```python
from build123d import *

# Parameters (mm, degrees)
EXTRUDE_1_DEPTH     = 36
SKETCH_2_R          = 1.05
CUT_EXTRUDE_1_DEPTH = 35
FILLET_1_R          = 1.5
FILLET_2_R          = 3
CUT_EXTRUDE_5_DEPTH = 50
SKETCH_5_W          = 24
SKETCH_5_H          = 86
SKETCH_5_R          = 5
EXTRUDE_2_DEPTH     = 1.5
SKETCH_6_W          = 2
SKETCH_6_H          = 6.336440046
CUT_EXTRUDE_6_DEPTH = 3.5
FILLET_3_R          = 1.5
FILLET_4_R          = 3
SKETCH_7_R          = 2.5
SKETCH_7_R_2        = 1.05
EXTRUDE_3_DEPTH     = 1.5
FILLET_5_R          = 1.5
CHAMFER_1_SIZE      = 2


with BuildPart() as part:
    # Эскиз1 → Вытянуть1 (new body)
    with BuildSketch(Plane.XY):
        Polygon((-20, 41.5), (0, 41.5), (0, 0), (36, 0), (36, 43.5), (60, 43.5), (60, 42), (37.5, 42), (37.5, -1.5), (-1.5, -1.5), (-1.5, 40), (-20, 40), align=None)
    extrude(amount=EXTRUDE_1_DEPTH)

    # Эскиз2 → Вырез-Вытянуть1 (cut)
    with BuildSketch(Plane(origin=(0, 41.5, 0), x_dir=(-1, 0, 0), z_dir=(0, 1, 0))):
        with Locations(Location((10, 5, 0), (0, 0, 90))):
            Circle(SKETCH_2_R)
        with Locations(Location((10, 31, 0), (0, 0, 90))):
            Circle(SKETCH_2_R)
    extrude(amount=-CUT_EXTRUDE_1_DEPTH, mode=Mode.SUBTRACT)

    # Скругление1
    fillet_1_edges = [part.edges().sort_by_distance(p)[0] for p in [
        (0, 0, 18),
        (36, 0, 18),
        (-1.5, 40, 18),
    ]]
    fillet(fillet_1_edges, radius=FILLET_1_R)

    # Скругление2
    fillet_2_edges = [part.edges().sort_by_distance(p)[0] for p in [
        (0, 41.5, 18),
        (37.5, -1.5, 18),
        (-1.5, -1.5, 18),
    ]]
    fillet(fillet_2_edges, radius=FILLET_2_R)

    # Эскиз4 → Вырез-Вытянуть5 (cut)
    with BuildSketch(Plane.ZY.offset(1.5)):
        Polygon((36, 0), (30.401923789, -1.5), (5.598076211, -1.5), (0, 0), (0, -9.726752533), (36, -8.93099636), align=None)
    extrude(amount=-CUT_EXTRUDE_5_DEPTH, mode=Mode.SUBTRACT)

    # Эскиз5 → Вытянуть2 (add)
    with BuildSketch(Plane(origin=(0, 43.5, 0), x_dir=(-1, 0, 0), z_dir=(0, 1, 0))):
        with Locations((-48, 18)):
            Rectangle(SKETCH_5_W, SKETCH_5_H)
        with Locations(Location((-48, -15, 0), (0, 0, 90))):
            Circle(SKETCH_5_R, mode=Mode.SUBTRACT)
        with Locations(Location((-48, 51, 0), (0, 0, 270))):
            Circle(SKETCH_5_R, mode=Mode.SUBTRACT)
    extrude(amount=-EXTRUDE_2_DEPTH)

    # Эскиз6 → Вырез-Вытянуть6 (cut)
    with BuildSketch(Plane.ZY.offset(-36)):
        with Locations((37, 42.938728947)):
            Rectangle(SKETCH_6_W, SKETCH_6_H)
        with Locations((-1, 42.938728947)):
            Rectangle(SKETCH_6_W, SKETCH_6_H)
    extrude(amount=-CUT_EXTRUDE_6_DEPTH, mode=Mode.SUBTRACT)

    # Скругление3
    fillet_3_edges = [part.edges().sort_by_distance(p)[0] for p in [
        (37.5, 42, 18),
    ]]
    fillet(fillet_3_edges, radius=FILLET_3_R)

    # Скругление4
    fillet_4_edges = [part.edges().sort_by_distance(p)[0] for p in [
        (36, 43.5, 18),
    ]]
    fillet(fillet_4_edges, radius=FILLET_4_R)

    # Эскиз7 → Вытянуть3 (add)
    # profile 1 of 2: a face of its own
    with BuildSketch(Plane.XZ.offset(-40)):
        with Locations(Location((-10, 31, 0), (0, 0, 90))):
            Circle(SKETCH_7_R)
        with Locations(Location((-10, 31, 0), (0, 0, 90))):
            Circle(SKETCH_7_R_2, mode=Mode.SUBTRACT)
    # profile 2 of 2: a face of its own
    with BuildSketch(Plane.XZ.offset(-40)):
        with Locations(Location((-10, 5, 0), (0, 0, 90))):
            Circle(SKETCH_7_R)
        with Locations(Location((-10, 5, 0), (0, 0, 90))):
            Circle(SKETCH_7_R_2, mode=Mode.SUBTRACT)
    extrude(amount=EXTRUDE_3_DEPTH)

    # Скругление5
    fillet_5_edges = [part.edges().sort_by_distance(p)[0] for p in [
        (-10, 40, 28.5),
        (-10, 40, 2.5),
        (-10, 41.5, 3.95),
        (-10, 41.5, 29.95),
    ]]
    fillet(fillet_5_edges, radius=FILLET_5_R - 0.0001)  # a hair under: the kernel refuses the full size

    # Фаска1
    chamfer_1_edges = [part.edges().sort_by_distance(p)[0] for p in [
        (36, 42.75, 61),
        (36, 42.75, -25),
        (60, 42.75, -25),
        (60, 42.75, 61),
    ]]
    chamfer(chamfer_1_edges, length=CHAMFER_1_SIZE)


solid = part.part
```
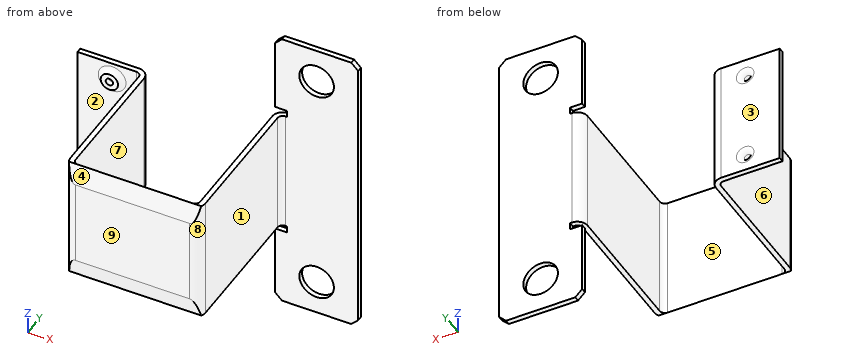
Source: CAD feature listing. Evaluate the final solid. Frame: model axes, mm. Face numbers are marked on the shaded views. A direction names the side the tool comes from. Coordinates: 2 decimals unless noted, no trailing zeros. Write each loop counter-clockwise with the first axis right and the second up, starting at its lowest first coordinate (ties: lowest second). Pieces come first, ordered by that corner, then holes. Notation, with made-up numbers: (-11.75, 75.5) -> (42.25, 75.5) arc R27 cw to (42.25, 99.5) -> close; hole circle Ø6 at (74, 1). An arc over 180 degrees is marked (long way). Return JSON: item names as keys, results as strings. Group by question number.
1) Section query A-A, the plane x = 48. Return loops of the section in (y, z).
2) Ray query, line 1 along X through (y, z) = (37, 18.5); line 2 along X through (y, z) = (39.55, 31); line 3 along X through (y, z) = (43.15, 51). Return the intervals inside material, ascending.
3) Mould query, pull axis X, two halves, no side actions, for the marked faces 6, 7, 8 and 9. Classes: +X half, -X half, draft (parallel to the pull), parting line (faces both ways), or undercut.
4) Section query D-D, the plane z = 15. Return loops of the section in (x, y).
5) Contact query for flat-ended pins moving along their axis: P1, Ø8, axis at y = 36.5, z = 17, coming from the +X side; P2, Ø1.6, axis at y = 42.5, z = -1.5, coming from the -X side; P3, Ø1.2, axis at x = 37.5, y = 43, coming from the -Z side; P4, Ø8.5, axis at x = -12.5, z = 21.5, coming from the -Y side. Output: stop coordinate, or through.
6) Section query C-C, the plane y = 17.5. Return loops of the section in (x, z).
7) Section query B-B, the plane z = -15. Return loops of the section in (x, y), plus the area to 3 significant figures.
8) Set-up query: the marked faces 1, 2, 3, 4 and 5. Return all of +Z, -Z, +X, -X, +Y, -Y with unobstructed straight access to the full face (end or side cutting, diameter ignored); none if empty.
From the geometry:
{
 "1": {"outline": "(42, -25) -> (43.5, -25) -> (43.5, -20) -> (42, -20) -> close; (42, -10) -> (43.5, -10) -> (43.5, 46) -> (42, 46) -> close; (42, 56) -> (43.5, 56) -> (43.5, 61) -> (42, 61) -> close"},
 "2": {"line 1": "-1.5 to 0, 36 to 37.5", "line 2": "-12.93 to -11.05, -8.95 to -7.07, -1.93 to -0.19, 36 to 37.5", "line 3": "36 to 43, 53 to 60"},
 "3": {"face 6": "-X half", "face 7": "undercut", "face 8": "+X half", "face 9": "draft"},
 "4": {"outline": "(-20, 40) -> (-3, 40) arc R1.5 cw to (-1.5, 38.5) -> (-1.5, 1.5) arc R3 ccw to (1.5, -1.5) -> (34.5, -1.5) arc R3 ccw to (37.5, 1.5) -> (37.5, 40.5) arc R1.5 cw to (39, 42) -> (60, 42) -> (60, 43.5) -> (39, 43.5) arc R3 ccw to (36, 40.5) -> (36, 1.5) arc R1.5 cw to (34.5, 0) -> (1.5, 0) arc R1.5 cw to (0, 1.5) -> (0, 38.5) arc R3 ccw to (-3, 41.5) -> (-20, 41.5) -> close"},
 "5": {"P1": "x = 37.5", "P2": "x = 36", "P3": "z = -25", "P4": "y = 40"},
 "6": {"outline": "(-1.5, 0) -> (0, 0) -> (0, 36) -> (-1.5, 36) -> close; (36, 0) -> (37.5, 0) -> (37.5, 36) -> (36, 36) -> close"},
 "7": {"outline": "(36, 42) -> (43, 42) -> (43, 43.5) -> (36, 43.5) -> close; (53, 42) -> (60, 42) -> (60, 43.5) -> (53, 43.5) -> close", "area": "21.0 mm²"},
 "8": {"face 1": "+Z, -Z, +X, -Y", "face 2": "-Y", "face 3": "+Z, -Z, -X, +Y", "face 4": "+Z, +X, -X, -Y", "face 5": "+Z, -Z, +Y"}
}
